```python
from build123d import *

# Parameters (mm, degrees)
CYLINDER_R        = 60
CYLINDER_DEPTH    = 5
CYLINDER001_R     = 53.5
CYLINDER001_DEPTH = 50
SKETCH001_R       = 51.3
POCKET_DEPTH      = 45


with BuildPart() as part:
    # Cylinder → Cylinder (join)
    with BuildSketch(Plane.XY):
        Circle(CYLINDER_R)
    extrude(amount=CYLINDER_DEPTH)

    # Cylinder001 → Cylinder001 (join)
    with BuildSketch(Plane.XY):
        Circle(CYLINDER001_R)
    extrude(amount=CYLINDER001_DEPTH)

    # Sketch001 (on Face6 of Cylinder001) → Pocket (cut)
    with BuildSketch(Plane.XY.offset(50)):
        Circle(SKETCH001_R)
    extrude(amount=-POCKET_DEPTH, mode=Mode.SUBTRACT)


solid = part.part
```
The listing builds one solid part. Answer for the finished solid, in the listing's coordinates (mm). A direction names the side the tool comes from. Give positions to 0.01 mm unless a question says otherwise; leave off trailing zeros. Order: outer loops, then holes, each group sorted by start corner. A loop starts at its lowest first (then second) coordinate and runs counter-clockwise, first axis right, second up.
1) Find section C-C on z = 10. Write down the section's boundary in (x, y).
Reported:
outline: circle Ø107 at (0, 0); hole circle Ø102.6 at (0, 0)
2) Consider line 1 along Y through (x, z) = (0, 17); line 2 along Z through (x, y) = (41, 39.5); line 3 along Y through (x, z) = (-41, 23.5). Determine where each line is inside the solid, lowest interval first.
Reported:
line 1: y = -53.5 to -51.3, 51.3 to 53.5
line 2: z = 0 to 5
line 3: y = -34.37 to -30.83, 30.83 to 34.37
3) For faces 1 (the face through (-54, 0, 5)), 2 (the face through (-4.2, -51.3, 50)), determine the directions among +Z, -Z, +X, -X, +Y, -Y from which every point of the face is accessible in a straight line to the end or side of a thin tool.
Reported:
face 1: +Z
face 2: +Z, +X, -X, +Y, -Y
4) Determine the mould class of faces 3 (the face through (-1, 1, 0)), 4 (the face through (-6.678, 50.863, 27.815)), 5 (the face through (-11.598, -52.228, 27.185)), 6 (the face through (-1, 1, 5)) for opening direction Y: pulls with the +Y half, pulls with the -Y half, needs draft (parallel to the pull), parting line crosses it, or undercut.
Reported:
face 3: needs draft
face 4: undercut
face 5: parting line crosses it
face 6: undercut
5) Given P1, Ø1.5, axis at x = 32.5, z = 41, coming from the -Y side; P2, Ø2, axis at x = -2.5, z = 40.5, coming from the +Y side; P3, Ø5, axis at x = -9.5, y = -20.5, coming from the +Z side; P4, Ø5, axis at x = 22, y = -5.5, coming from the -Z side, each flat-ended and moving along its own axis, determine where each tip first touches the part or whether it passes through.
Reported:
P1: stops at y = -43.06
P2: stops at y = 53.48
P3: stops at z = 5
P4: stops at z = 0
6) Find section A-A on y = 0. Write down the section's boundary in (x, z), then the cut area to 3 significant figures.
Reported:
outline: (-60, 0) - (60, 0) - (60, 5) - (53.5, 5) - (53.5, 50) - (51.3, 50) - (51.3, 5) - (-51.3, 5) - (-51.3, 50) - (-53.5, 50) - (-53.5, 5) - (-60, 5) - close
area: 798 mm2
